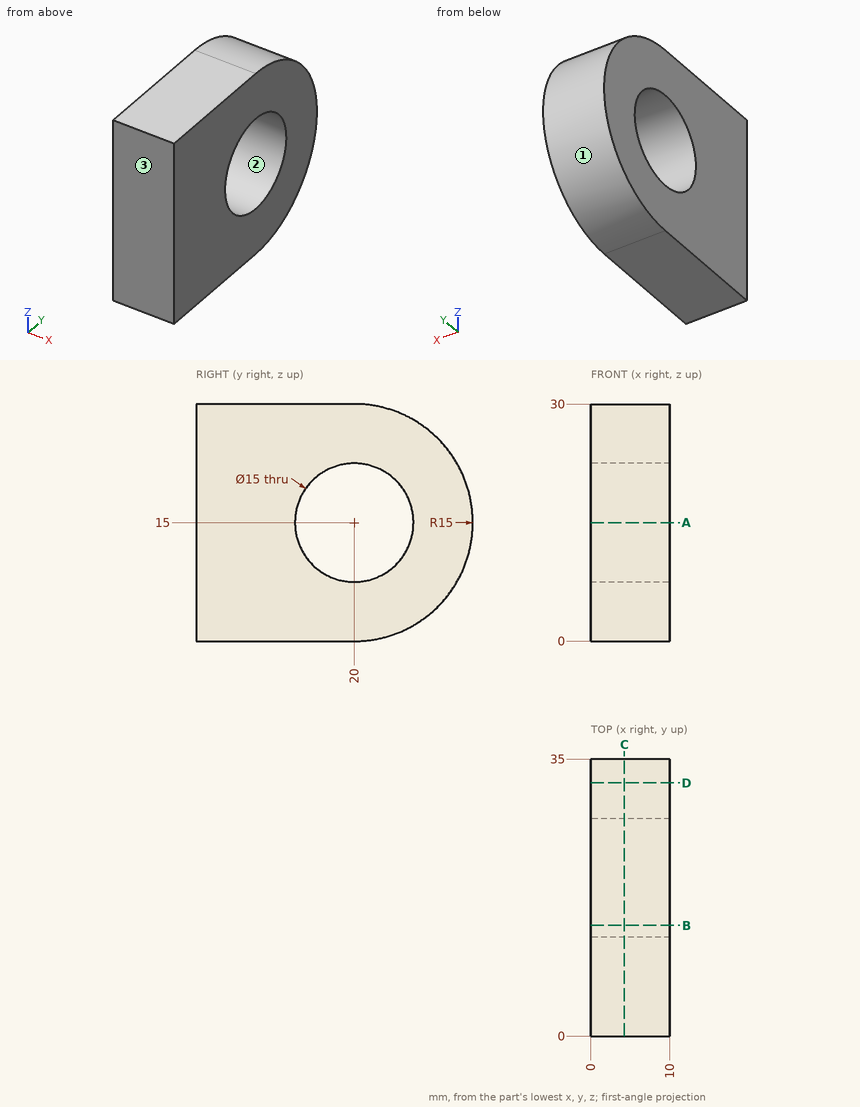
Geometry check sheet. Reference: drawing and pictorial views, mm from the part's lowest x, y, z. Coordinates: 2 decimals unless noted, no trailing zeros. Order: outer loops, then holes, each group sorted by start corner. A loop starts at its lowest first (then second) coordinate and runs counter-clockwise, first axis right, second up.
Item 1: Section check A-A, the plane z = 15. Enter the section's corners in (x, y).
Filled in:
outline: (0, 0) - (10, 0) - (10, 12.5) - (0, 12.5) - close; (0, 27.5) - (10, 27.5) - (10, 35) - (0, 35) - close
Item 2: Depth check by flat-ended pin: pin 1 (2 mm diameter, centred on x = 2.5, y = 27, fed in from +Z); pin 2 (3 mm diameter, centred on x = 1, z = 23.5, fed in from +Y). Enter the tip coordinate at first touch or a pass-through.
Filled in:
pin 1: stops at z = 28.75
pin 2: stops at y = 33.27
Item 3: Material ranges on L1, parallel to Y at x = 2.5, z = 15; L2, parallel to Z at x = 4, y = 26; L3, parallel to Y at x = 3.5, z = 9, recorded low to high.
Filled in:
L1: y = 0 to 12.5, 27.5 to 35
L2: z = 1.25 to 10.5, 19.5 to 28.75
L3: y = 0 to 15.5, 24.5 to 33.75
Item 4: Section check C-C, the plane x = 4.25. Enter the section's corners in (y, z).
Filled in:
outline: (0, 0) - (20, 0) arc R15 ccw to (20, 30) - (0, 30) - close; hole circle Ø15 at (20, 15)
Item 5: Section check B-B, the plane y = 14. Enter the section's corners in (x, z).
Filled in:
outline: (0, 0) - (10, 0) - (10, 10.5) - (0, 10.5) - close; (0, 19.5) - (10, 19.5) - (10, 30) - (0, 30) - close
Item 6: Release check for a two-part mould opening along Z. For the marked faces 1, 2 and 3 record: +Z half, -Z half, draft (parallel to the pull), parting line (faces both ways), or undercut.
Filled in:
face 1: parting line
face 2: undercut
face 3: draft
Item 7: Section check D-D, the plane y = 32. Enter the section's corners in (x, z), then the cut area to 3 significant figures.
Filled in:
outline: (0, 6) - (10, 6) - (10, 24) - (0, 24) - close
area: 180 mm2
